from build123d import *

# Parameters (mm, degrees)
F0_W           = 5
F0_H           = 5.5
F0_W_2         = 5.5
F0_H_2         = 5
F0_W_3         = 51
F0_H_3         = 51
F1_DEPTH       = 190
F2_R           = 10
F4_D           = 5.1054
F4_DEPTH       = 12
F4_CSINK_D     = 10.4394
F4_CSINK_ANGLE = 82
F4_TIP         = 1.5338169022
F6_D           = 5.1054
F6_DEPTH       = 12
F6_CSINK_D     = 10.4394
F6_CSINK_ANGLE = 82
F6_TIP         = 1.5338169022


with BuildPart() as f1:
    # F0 (on Top) → F1 (new body)
    with BuildSketch(Plane.XY):
        Polygon((-33.5, 28), (-28, 28), (-28, 33.5), (-28, 36.5), (-36.5, 36.5), (-36.5, 28), align=None)
        Polygon((-28, 36.5), (-28, 33.5), (-23, 33.5), (-13, 33.5), (-13, 36.5), align=None)
        with Locations((-25.5, 30.75)):
            Rectangle(F0_W, F0_H)
        with Locations((-30.75, 25.5)):
            Rectangle(F0_W_2, F0_H_2)
        Polygon((-33.5, 23), (-33.5, 28), (-36.5, 28), (-36.5, 13), (-33.5, 13), align=None)
        Polygon((-23, 28), (-28, 28), (-28, 23), (-28, -30.5), (30.5, -30.5), (30.5, 28), align=None)
        Rectangle(F0_W_3, F0_H_3, mode=Mode.SUBTRACT)
    extrude(amount=F1_DEPTH)

    # F2
    f2_edges = [f1.edges().sort_by_distance(p)[0] for p in [
        (-36.5, 36.5, 95),
    ]]
    fillet(f2_edges, radius=F2_R)

    # F4
    with Locations(Plane.XZ.offset(30.5)):
        with Locations((0, 140), (0, 60)):
            CounterSinkHole(F4_D / 2, F4_CSINK_D / 2, depth=F4_DEPTH, counter_sink_angle=F4_CSINK_ANGLE)
            with Locations((0, 0, -(F4_DEPTH + F4_TIP / 2))):  # 118° drill point
                Cone(0, F4_D / 2, F4_TIP, mode=Mode.SUBTRACT)

    # F6
    with Locations(Plane.YZ.offset(30.5)):
        with Locations((0, 130), (0, 50)):
            CounterSinkHole(F6_D / 2, F6_CSINK_D / 2, depth=F6_DEPTH, counter_sink_angle=F6_CSINK_ANGLE)
            with Locations((0, 0, -(F6_DEPTH + F6_TIP / 2))):  # 118° drill point
                Cone(0, F6_D / 2, F6_TIP, mode=Mode.SUBTRACT)


solid = f1.part
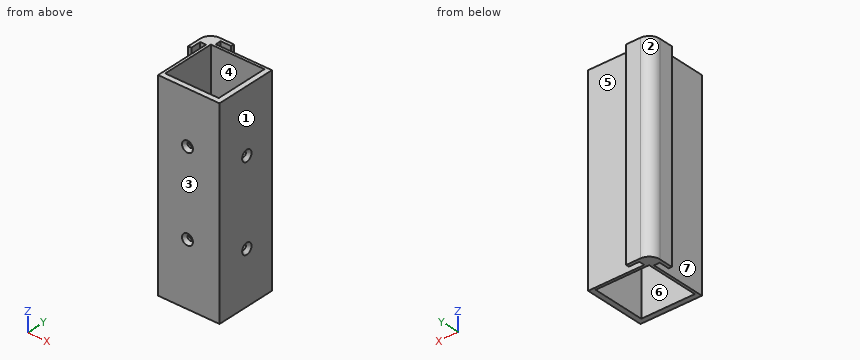
The model under review builds one solid part; all positions refer to its coordinate system, in mm. Face numbers are marked on the shaded views. A direction names the side the tool comes from. Give positions to 0.01 mm unless a question says otherwise; leave off trailing zeros. Order: outer loops, then holes, each group sorted by start corner. A loop starts at its lowest first (then second) coordinate and runs counter-clockwise, first axis right, second up. Notation, with made-up numbers: M -7.5,-32 L 21.5,-32 A12 cw 21.5,-24 Z; hole C 28.5,-7.5 d3. An arc over 180 degrees is marked long. Answer in a Markdown table with one row per item. Add a question column.
1. Add section C-C on y = 0. State the section outline as (x, z) points.
2. To check wall thickness, follow line 1 along X through (y, z) = (18, 26.5); line 2 along Y through (x, z) = (-17.5, 126.5); line 3 along X through (y, z) = (-24.5, 36.5). State the ranges of each line that lie inside material, in increasing order.
3. Add section A-A on z = 81. State the section outline as (x, y) points, plus the area to 3 significant figures.
4. For pin 1 Ø4 at (y, z) = (-10, 57) entering from -X; pin 2 Ø6 at (x, z) = (0, 140) entering from +Y; pin 3 Ø4.5 at (y, z) = (30, 99) entering from +X; pin 4 Ø1.5 at (y, z) = (35, 115) entering from +X, all flat-tipped, find the tip position at first contact; note any pin that passes through.
5. Mouldability with a two-part tool opening along Y and no side actions: class the marked faces 1, 2, 3 and 4 as released by +Y, released by -Y, zero draft, split by the parting line, or undercut.
6. Add section D-D on x = -10.5. State the section outline as (y, z) points, plus the area to 4 significant figures.
7. Machinability: for the marked faces 5, 6 and 7, which of the approach directions +Z, -Z, +X, -X, +Y, -Y give a long, thin tool a straight path to every point of the face, cutting with its end or side? Answer none if there is none.
8. Add section B-B on x = 0. State the section outline as (y, z) points.
The answers:
| question | item | result |
|---|---|---|
| 1 | outline | M -28,0 L -25.5,0 L -25.5,190 L -28,190 Z; M 25.5,0 L 30.5,0 L 30.5,44.78 L 27.43,47.45 L 25.5,47.45 Z; M 25.5,52.55 L 27.43,52.55 L 30.5,55.22 L 30.5,124.78 L 27.43,127.45 L 25.5,127.45 Z; M 25.5,132.55 L 27.43,132.55 L 30.5,135.22 L 30.5,190 L 25.5,190 Z |
| 2 | line 1 | -36.5 to -33.5, -28 to -25.5, 25.5 to 30.5 |
| 2 | line 2 | -30.5 to -25.5, 25.5 to 28, 33.5 to 36.5 |
| 2 | line 3 | -28 to -25.5, 25.5 to 30.5 |
| 3 | outline | M -36.5,13 L -33.5,13 L -33.5,23 L -28,23 L -28,-30.5 L 30.5,-30.5 L 30.5,28 L -23,28 L -23,33.5 L -13,33.5 L -13,36.5 L -26.5,36.5 A10 ccw -36.5,26.5 Z; hole M -25.5,-25.5 L 25.5,-25.5 L 25.5,25.5 L -25.5,25.5 Z |
| 3 | area | 1,020 mm2 |
| 4 | pin 1 | x = -28 |
| 4 | pin 2 | y = 28 |
| 4 | pin 3 | x = 30.5 |
| 4 | pin 4 | x = -13 |
| 5 | face 1 | zero draft |
| 5 | face 2 | released by +Y |
| 5 | face 3 | released by -Y |
| 5 | face 4 | undercut |
| 6 | outline | M -30.5,0 L -25.5,0 L -25.5,190 L -30.5,190 Z; M 25.5,0 L 28,0 L 28,190 L 25.5,190 Z |
| 6 | area | 1,425 mm2 |
| 7 | face 5 | +Z, -Z, +X |
| 7 | face 6 | +Z, -Z |
| 7 | face 7 | +Z, -Z, -Y |
| 8 | outline | M -30.5,0 L -25.5,0 L -25.5,57.45 L -27.43,57.45 L -30.5,54.78 Z; M -30.5,65.22 L -27.43,62.55 L -25.5,62.55 L -25.5,137.45 L -27.43,137.45 L -30.5,134.78 Z; M -30.5,145.22 L -27.43,142.55 L -25.5,142.55 L -25.5,190 L -30.5,190 Z; M 25.5,0 L 28,0 L 28,190 L 25.5,190 Z |
